from build123d import *

# Parameters (mm, degrees)
F0_W     = 28
F0_H     = 28
F1_DEPTH = 16
F3_D     = 4
F4_DEPTH = 3


with BuildPart() as f1:
    # F0 (on Top) → F1 (new body)
    with BuildSketch(Plane.XY):
        Rectangle(F0_W, F0_H)
    extrude(amount=F1_DEPTH)

    # F3 (through all)
    with Locations(Plane.XY.offset(16)):
        with Locations((4, -6.5), (-6.5, -6.5), (-6.5, 6.5), (4, 6.5)):
            Hole(F3_D / 2)

    # F4 (cut): a face of the model
    f4_faces = [f1.faces().sort_by_distance(p)[0] for p in [
        (14, 0, 8),
    ]]
    extrude(f4_faces, amount=-F4_DEPTH, mode=Mode.SUBTRACT)


solid = f1.part
Geometry: final body of the model. Coordinates: model frame, mm. Round coordinates to 2 decimals unless told otherwise and drop trailing zeros. Order: outer loops, then holes, each group sorted by start corner. A loop starts at its lowest first (then second) coordinate and runs counter-clockwise, first axis right, second up. Notation, with made-up numbers: (59.25, 27) - (67.25, 27) arc R30 cw to (67.25, 58) - close; hole circle Ø10 at (60, -38.75). An arc over 180 degrees is marked (long way). Write each question's results on one line, items separated by ' | '.
Item 1: Section C-C, the plane x = -6.5. Return the cut outline in (y, z).
Completed:
outline: (-14, 0) - (-8.5, 0) - (-8.5, 16) - (-14, 16) - close; (-4.5, 0) - (4.5, 0) - (4.5, 16) - (-4.5, 16) - close; (8.5, 0) - (14, 0) - (14, 16) - (8.5, 16) - close
Item 2: First-contact query: pin 1 Ø4.5 at (x, y) = (-6.5, -6.5) entering from +Z; pin 2 Ø2.5 at (x, y) = (-6.5, 6.5) entering from +Z. Flat tips, straight axial feed; report the tip coordinate or a pass-through.
Completed:
pin 1: z = 16 | pin 2: through
Item 3: Section A-A, the plane y = -6.5. Return the cut outline in (x, z), and give its area (3 significant figures).
Completed:
outline: (-14, 0) - (-8.5, 0) - (-8.5, 16) - (-14, 16) - close; (-4.5, 0) - (2, 0) - (2, 16) - (-4.5, 16) - close; (6, 0) - (11, 0) - (11, 16) - (6, 16) - close | area: 272 mm^2
Item 4: Material intervals for line 1 along Y through (x, z) = (-6.5, 9.5); line 2 along X through (y, z) = (5, 10.25); line 3 along X through (y, z) = (-7.25, 13.5), sorted ascending. Write a range as [from, to].
Completed:
line 1: [-14, -8.5], [-4.5, 4.5], [8.5, 14] | line 2: [-14, -7.82], [-5.18, 2.68], [5.32, 11] | line 3: [-14, -8.35], [-4.65, 2.15], [5.85, 11]
Item 5: Section B-B, the plane z = 14.25. Return the cut outline in (x, y).
Completed:
outline: (-14, -14) - (11, -14) - (11, 14) - (-14, 14) - close; hole circle Ø4 at (-6.5, -6.5); hole circle Ø4 at (-6.5, 6.5); hole circle Ø4 at (4, -6.5); hole circle Ø4 at (4, 6.5)
Item 6: Mould query, pull axis Y, two halves, no side actions, for faces 1 (the flat face through (-2, 0, 16)), 2 (the flat face through (-2, 14, 8)), 3 (the cylindrical face through (5.6, -7.7, 7.9)). Classes: pulls with the +Y half, pulls with the -Y half, needs draft (parallel to the pull), parting line crosses it, or undercut.
Completed:
face 1: needs draft | face 2: pulls with the +Y half | face 3: undercut
